The listing builds one solid part. Answer for the finished solid, in the listing's coordinates (mm). Face numbers are marked on the shaded views. A direction names the side the tool comes from. Round coordinates to 2 decimals unless told otherwise and drop trailing zeros. Write each loop counter-clockwise with the first axis right and the second up, starting at its lowest first coordinate (ties: lowest second). Pieces come first, ordered by that corner, then holes. Notation, with made-up numbers: M -30,26.25 L -26,26.25 A16 cw -26,43.25 Z; hole C 43,32 d10. An arc over 180 degrees is marked long. Write each question's results on one line, items separated by ' | '.
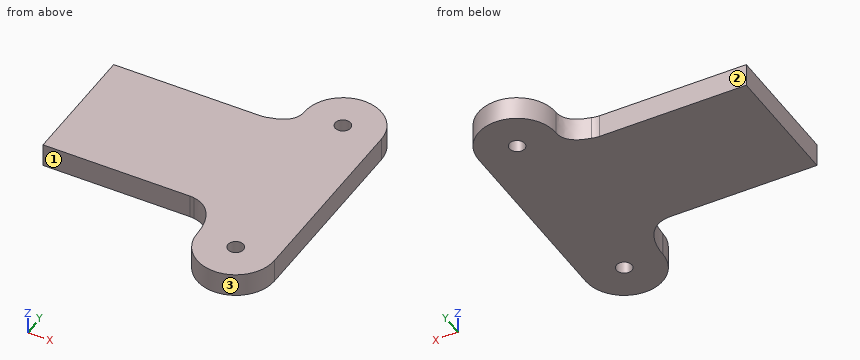
from build123d import *

# Parameters (mm, degrees)
SKETCH1_R           = 1
BOSS_EXTRUDE1_DEPTH = 3
SKETCH5_OUTSIDE_W   = 34.508
SKETCH5_OUTSIDE_H   = 45.508
SKETCH5_OUTSIDE_R   = 1
CUT_EXTRUDE2_DEPTH  = 10
SKETCH7_W           = 3
SKETCH7_H           = 10
SKETCH7_H_2         = 4
BOSS_EXTRUDE2_DEPTH = 10
BOSS_EXTRUDE3_REACH = 32.956
SKETCH8_W           = 22
SKETCH8_H           = 3


with BuildPart() as part:
    # Sketch1 → Boss-Extrude1 (new body)
    with BuildSketch(Plane.XY):
        with BuildLine():
            Line((0, 0), (0, -10))
            Line((0, -10), (9, -10))
            ThreePointArc((9, -10), (11.121320344, -10.878679656), (12, -13))
            Line((12, -13), (12, -17.5))
            ThreePointArc((12, -17.5), (12.878679656, -19.621320344), (15, -20.5))
            Line((15, -20.5), (21, -20.5))
            ThreePointArc((21, -20.5), (23.121320344, -19.621320344), (24, -17.5))
            Line((24, -17.5), (24, 11.5))
            ThreePointArc((24, 11.5), (23.121320344, 13.621320344), (21, 14.5))
            Line((21, 14.5), (15, 14.5))
            ThreePointArc((15, 14.5), (12.878679656, 13.621320344), (12, 11.5))
            Line((12, 11.5), (12, 9.5))
            ThreePointArc((12, 9.5), (11.121320344, 7.378679656), (9, 6.5))
            Line((9, 6.5), (0, 6.5))
            Line((0, 6.5), (0, 2.5))
            Line((0, 2.5), (12, 2.5))
            Line((12, 2.5), (12, 0))
            Line((12, 0), (0, 0))
        make_face()
        with Locations((18, -15.5)):
            Circle(SKETCH1_R, mode=Mode.SUBTRACT)
        with Locations((18, 9.5)):
            Circle(SKETCH1_R, mode=Mode.SUBTRACT)
    extrude(amount=BOSS_EXTRUDE1_DEPTH)

    # Sketch5 outside → Cut-Extrude2 (cut)
    # profile 1 of 3: a face of its own
    with BuildSketch(Plane.XY.offset(3)):
        with Locations((12, -3)):
            Rectangle(SKETCH5_OUTSIDE_W, SKETCH5_OUTSIDE_H)
        with BuildLine():
            Line((23, -15.5), (23, 9.5))
            ThreePointArc((23, 9.5), (18, 14.5), (13, 9.5))
            ThreePointArc((13, 9.5), (13.00003125, 9.482322297), (13.000125, 9.464644815))
            add(Edge.make_bspline(
                [(9.978094602, 6.663923317), (12.995350289, 7.319865218), (13.000125, 9.464644815)],
                knots=[0.130065152, 0.130065152, 0.130065152, 0.992908545, 0.992908545, 0.992908545], degree=2))
            ThreePointArc((9.978094602, 6.663923317), (9.495867902, 6.541264624), (9, 6.5))
            Line((9, 6.5), (0, 6.5))
            Line((0, 6.5), (0, 2.5))
            Line((0, 2.5), (12, 2.5))
            Line((12, 2.5), (12, 0))
            Line((12, 0), (0, 0))
            Line((0, 0), (0, -10))
            Line((0, -10), (9, -10))
            ThreePointArc((9, -10), (9.288075976, -10.013863327), (9.573489492, -10.055325179))
            add(Edge.make_bspline(
                [(13.000670773, -15.418101992), (13.007397522, -13.305169489), (12.200422908, -10.491068866), (9.573489492, -10.055325179)],
                knots=[0.011989502, 0.011989502, 0.011989502, 0.011989502, 0.935888971, 0.935888971, 0.935888971, 0.935888971], degree=3))
            add(Edge.make_bspline(
                [(13, -15.5), (13.000359156, -15.47282323), (13.00058348, -15.445521651), (13.000670773, -15.418101992)],
                knots=[0, 0, 0, 0, 0.011989502, 0.011989502, 0.011989502, 0.011989502], degree=3))
            ThreePointArc((13, -15.5), (18, -20.5), (23, -15.5))
        make_face(mode=Mode.SUBTRACT)
    # profile 2 of 3: a face of its own
    with BuildSketch(Plane.XY.offset(3)):
        with Locations((18, -15.5)):
            Circle(SKETCH5_OUTSIDE_R)
    # profile 3 of 3: a face of its own
    with BuildSketch(Plane.XY.offset(3)):
        with Locations((18, 9.5)):
            Circle(SKETCH5_OUTSIDE_R)
    extrude(amount=-CUT_EXTRUDE2_DEPTH, mode=Mode.SUBTRACT)

    # Sketch7 → Boss-Extrude2 (add)
    with BuildSketch(Plane.ZY):
        with Locations((1.5, -5)):
            Rectangle(SKETCH7_W, SKETCH7_H)
        with Locations((1.5, 4.5)):
            Rectangle(SKETCH7_W, SKETCH7_H_2)
    extrude(amount=BOSS_EXTRUDE2_DEPTH)

    # Sketch8 → Boss-Extrude3 (add, up to next)
    with BuildSketch(Plane(origin=(0, 0, 0), x_dir=(1, 0, 0), z_dir=(0, 1, 0)), mode=Mode.PRIVATE) as boss_extrude3_sk1:
        with Locations((1, -1.5)):
            Rectangle(SKETCH8_W, SKETCH8_H)
    boss_extrude3_tool1 = extrude(boss_extrude3_sk1.sketch, amount=BOSS_EXTRUDE3_REACH, mode=Mode.PRIVATE) - part.part
    add(boss_extrude3_tool1.solids().sort_by_distance((1, 0, 1.5))[0])


solid = part.part
1) Section D-D (y = 11.5) is taken. Determine the outline of the cut face in (x, z), then the cut area to 3 significant figures.
Return value:
outline: M 13.42,0 L 22.58,0 L 22.58,3 L 13.42,3 Z | area: 27.5 mm²
2) Section B-B (z = 2.35) is taken. State how many separate pieces and enclosed holes the cut face has, then the cut area to 3 significant figures.
Return value:
separate pieces: 1 | enclosed holes: 2 | area: 709 mm²
3) Find the intervals of material crossed by line 1 (Y direction, x = 18, z = 0.75); line 2 (Y direction, x = -7, z = 1.35); line 3 (Y direction, x = 21, z = 0.3), in increasing order.
Return value:
line 1: -20.5 to -16.5, -14.5 to 8.5, 10.5 to 14.5 | line 2: -10 to 6.5 | line 3: -19.5 to 13.5
4) Each of these flat-tipped pins is pushed along its axis until it touches: pin 1 (1 mm diameter, centred on x = -4.5, z = 0.5, fed in from +Y); pin 2 (1 mm diameter, centred on x = -2.5, z = 0.5, fed in from -Y). Where does it stop, or does it pass through?
Return value:
pin 1: y = 6.5 | pin 2: y = -10
5) Section C-C (x = 4) is taken. Determine the outline of the cut face in (y, z), then the cut area to 3 significant figures.
Return value:
outline: M -10,0 L 6.5,0 L 6.5,3 L -10,3 Z | area: 49.5 mm²
6) A tool of negligible diameter and unlimited length cuts with its end or side. For the marked faces 1, 2 and 3, from which of +Z, -Z, +X, -X, +Y, -Y can it reach the whole face along a straight path? Write none if from no direction.
Return value:
face 1: +Z, -Z, -X, -Y | face 2: +Z, -Z, -X, +Y | face 3: +Z, -Z, -Y
7) Section A-A (x = 18) is taken. Determine the outline of the cut face in (y, z).
Return value:
outline: M -20.5,0 L -16.5,0 L -16.5,3 L -20.5,3 Z; M -14.5,0 L 8.5,0 L 8.5,3 L -14.5,3 Z; M 10.5,0 L 14.5,0 L 14.5,3 L 10.5,3 Z
